Check sheet for the modelled part. Datum: model origin and axes. Units: mm. Face numbers are marked on the shaded views. A direction names the side the tool comes from. Give positions to 0.01 mm unless a question says otherwise; leave off trailing zeros. Loops run counter-clockwise (first coordinate to the right, second up) from the corner with the lowest first, then second, coordinate; pieces in that order, holes last. Notation, with made-up numbers: (49.25, 53.5) - (70.25, 53.5) arc R30 ccw to (70.25, 87.5) - close; hole circle Ø7 at (4.5, -17). An arc over 180 degrees is marked (long way). Use CSV: the item, a comma, the result in double quotes.
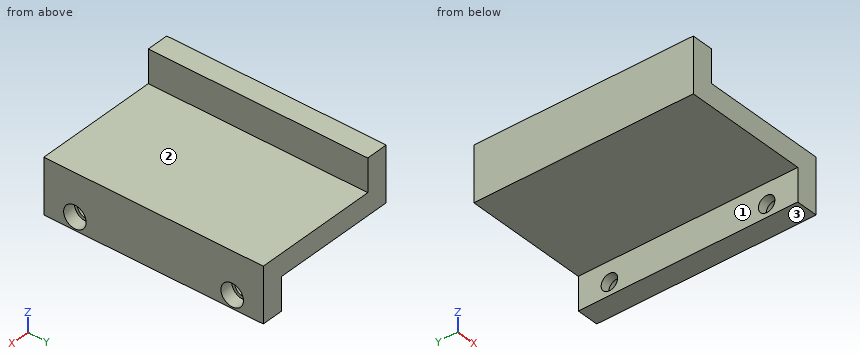
from build123d import *

# Parameters (mm, degrees)
F0_W     = 40
F0_H     = 60
F1_DEPTH = 24
F2_W     = 65.936946
F2_H     = 73.230896
F3_DEPTH = 9
F4_W     = 66.143565
F4_H     = 69.968968
F5_DEPTH = 9
F6_R     = 2.25
F7_DEPTH = 8
F8_R     = 3.075
F9_DEPTH = 3.5


with BuildPart() as f1:
    # F0 (on Top) → F1 (new body)
    with BuildSketch(Plane.XY):
        Rectangle(F0_W, F0_H)
    extrude(amount=F1_DEPTH)

    # F2 (on face) → F3 (cut)
    with BuildSketch(Plane.XY.offset(24)):
        with Locations((18.968473, 0)):
            Rectangle(F2_W, F2_H)
    extrude(amount=-F3_DEPTH, mode=Mode.SUBTRACT)

    # F4 (on face) → F5 (cut)
    with BuildSketch(Plane(origin=(0, 0, 0), x_dir=(1, 0, 0), z_dir=(0, 0, -1))):
        with Locations((-19.071782, 0)):
            Rectangle(F4_W, F4_H)
    extrude(amount=-F5_DEPTH, mode=Mode.SUBTRACT)

    # F6 (on face) → F7 (cut)
    with BuildSketch(Plane.YZ.offset(20)):
        with Locations((21.5, 3.5)):
            Circle(F6_R)
        with Locations((-21.5, 3.5)):
            Circle(F6_R)
    extrude(amount=-F7_DEPTH, mode=Mode.SUBTRACT)

    # F8 (on face) → F9 (cut)
    with BuildSketch(Plane.YZ.offset(20)):
        with Locations((-21.5, 3.5)):
            Circle(F8_R)
        with Locations((21.5, 3.5)):
            Circle(F8_R)
    extrude(amount=-F9_DEPTH, mode=Mode.SUBTRACT)


solid = f1.part
1. Go/stop test with flat-tipped pins: pin 1 Ø6 at (y, z) = (-19, 4.5) entering from -X; pin 2 Ø3 at (y, z) = (-22, 4.5) entering from +X; pin 3 Ø7 at (y, z) = (-13, 20) entering from +X. Record where each tip stops, or that it passes through.
Completed:
pin 1,"stops at x = 14"
pin 2,"stops at x = 16.5"
pin 3,"stops at x = -14"
2. Sectioned sample at D-D, the plane z = 8. Record the boundary of the cut face in (x, y).
Completed:
outline,"(14, -30) - (20, -30) - (20, 30) - (14, 30) - close"
3. Scan lines: line 1 along Y through (x, z) = (18, 6.25); line 2 along Z through (x, y) = (18.3, 21.5) (3 decimals); line 3 along X through (y, z) = (-11.5, 17). Record each from-to range of solid material in increasing order.
Completed:
line 1,"y = -30 to -22.88, -20.12 to 20.12, 22.88 to 30"
line 2,"z = 0 to 0.425, 6.575 to 15"
line 3,"x = -20 to -14"
4. Sectioned sample at C-C, the plane x = -16.5. Record the boundary of the cut face in (y, z).
Completed:
outline,"(-30, 9) - (30, 9) - (30, 24) - (-30, 24) - close"
5. Sectioned sample at A-A, the plane y = -21.5. Record the boundary of the cut face in (x, z) (3 decimals).
Completed:
outline,"(-20, 9) - (14, 9) - (14, 5.75) - (16.5, 5.75) - (16.5, 6.575) - (20, 6.575) - (20, 15) - (-14, 15) - (-14, 24) - (-20, 24) - close; (14, 0) - (20, 0) - (20, 0.425) - (16.5, 0.425) - (16.5, 1.25) - (14, 1.25) - close"
6. Set-up check for the marked faces 1, 2 and 3: record each of +Z, -Z, +X, -X, +Y, -Y from which the full face is reachable in a straight line by a thin tool's end or side.
Completed:
face 1,"-Z, -X, +Y, -Y"
face 2,"+Z, +X, +Y, -Y"
face 3,"-Z, +X, -X, +Y, -Y"
7. Sectioned sample at B-B, the plane z = 3.5. Record the boundary of the cut face in (x, y) (3 decimals), and give its area (3 significant figures).
Completed:
outline,"(14, -30) - (20, -30) - (20, -24.575) - (16.5, -24.575) - (16.5, -23.75) - (14, -23.75) - close; (14, -19.25) - (16.5, -19.25) - (16.5, -18.425) - (20, -18.425) - (20, 18.425) - (16.5, 18.425) - (16.5, 19.25) - (14, 19.25) - close; (14, 23.75) - (16.5, 23.75) - (16.5, 24.575) - (20, 24.575) - (20, 30) - (14, 30) - close"
area,"294 mm²"
